Autodesk Inventor part; units mm, degrees
ref_plane "YZ Plane" through (0, 0, 0) normal (1, 0, 0) x (0, 1, 0)
ref_plane "XZ Plane" through (0, 0, 0) normal (0, 1, 0) x (-1, 0, 0)
ref_plane "XY Plane" through (0, 0, 0) normal (0, 0, 1) x (1, 0, 0)
sketch "スケッチ2" plane through (0, 0, 0) normal (0, 1, 0) x (-1, 0, 0)
  line L0 (-6, 0) -> (-6, 5)
  line L1 (-6, 5) -> (-10, 5)
  line L2 (-10, 5) -> (-10, 11.5)
  line L3 (-10, 11.5) -> (-6, 11.5)
  line L4 (-6, 11.5) -> (-6, 12.5)
  line L5 (-6, 12.5) -> (-4, 12.5)
  line L6 (-4, 12.5) -> (-4, 0)
  line L7 (-4, 0) -> (-6, 0)
  line L8 (0, -14.5) -> (0, 17)
  circle A0 centre (0, 0) radius 4 construction
  circle A1 centre (0, 0) radius 10 construction
  circle A2 centre (0, 0) radius 6.7 construction
  dimension "d4" = 4
  dimension "d5" = 6
  dimension "d6" = 10
  dimension "d7" = 12.5
  dimension "d8" = 5
  dimension "d9" = 1
  dimension "d11" = 8
  dimension "d12" = 20
  dimension "d14" = 3.3
revolve "回転1" add sketch "スケッチ2" angle 360 about axis through (0, 0, -10) along (0, 0, 1)
mirror "ミラー1" about plane through (6, 0, 0) normal (0, 0, -1) of "回転1"
properties part number "POMベアリング" material "アセタール樹脂、白"
Build history of the part. All positions in model axes, mm. A direction names the side the tool comes from. Round coordinates to 2 decimals unless told otherwise and drop trailing zeros. Loops run counter-clockwise (first coordinate to the right, second up) from the corner with the lowest first, then second, coordinate; pieces in that order, holes last. Notation, with made-up numbers: (14.25, 33) -> (21.25, 33) arc R5 cw to (21.25, 41) -> close; hole circle Ø9 at (76.25, -10). An arc over 180 degrees is marked (long way). Answer in a Markdown table with one row per item.
Item 1: Pin check, flat tips, straight feed: pin 1 (1.5 mm diameter, centred on x = -7.5, z = -5, fed in from -Y); pin 2 (1.5 mm diameter, centred on x = 1.5, z = 9.5, fed in from +Y); pin 3 (2 mm diameter, centred on x = -2, z = -3, fed in from -Y); pin 4 (7 mm diameter, centred on x = 0, y = 0, fed in from +Z). Stop position of each tip, or through.
Answers below:
| item | result |
|---|---|
| pin 1 | stops at y = -7.38 |
| pin 2 | stops at y = 9.97 |
| pin 3 | stops at y = -5.92 |
| pin 4 | passes through |
Item 2: Mould opens along Z. For faces 1 (the flat face through (7, 0, 5)), 2 (the cylindrical face through (-0.867, -3.905, 0.175)), 3 (the flat face through (-1.42, -3.92, 12.5)) say: +Z half, -Z half, draft (parallel to the pull), parting line (faces both ways), or undercut.
Answers below:
| item | result |
|---|---|
| face 1 | undercut |
| face 2 | draft |
| face 3 | +Z half |
Item 3: Saw through at A-A (y = 0). Write the cut outline in (x, z), and give its area (3 significant figures).
Answers below:
| item | result |
|---|---|
| outline | (-10, -11.5) -> (-6, -11.5) -> (-6, -12.5) -> (-4, -12.5) -> (-4, 12.5) -> (-6, 12.5) -> (-6, 11.5) -> (-10, 11.5) -> (-10, 5) -> (-6, 5) -> (-6, -5) -> (-10, -5) -> close; (4, -12.5) -> (6, -12.5) -> (6, -11.5) -> (10, -11.5) -> (10, -5) -> (6, -5) -> (6, 5) -> (10, 5) -> (10, 11.5) -> (6, 11.5) -> (6, 12.5) -> (4, 12.5) -> close |
| area | 204 mm² |
Item 4: Saw through at C-C (z = 10.5). Write the cut outline in (x, y), and give its area (3 significant figures).
Answers below:
| item | result |
|---|---|
| outline | circle Ø20 at (0, 0); hole circle Ø8 at (0, 0) |
| area | 264 mm² |
Item 5: Drill centre lines: L1, parallel to Z at x = 8, y = 1; L2, parallel to Y at x = 0, z = -5.25; L3, parallel to Y at x = 0, z = 1.5. Where is each one in solid material? Low to high. Write a range as [from, to].
Answers below:
| item | result |
|---|---|
| L1 | z = [-11.5, -5], [5, 11.5] |
| L2 | y = [-10, -4], [4, 10] |
| L3 | y = [-6, -4], [4, 6] |
Item 6: Which spindle directions (+Z, -Z, +X, -X, +Y, -Y) get a long thin tool onto all of the face, cutting with end or side? Do faces 4 (the cylindrical face through (-6, 0, -12)), 5 (the cylindrical face through (-6, 0, 0)), 6 (the flat face through (1.42, -3.92, -12.5)), 7 (the cylindrical face through (-6, 0, 12)), 8 (the cylindrical face through (-2.17, -9.76, 8.3)). Say none if no direction does.
Answers below:
| item | result |
|---|---|
| face 4 | -Z |
| face 5 | none |
| face 6 | -Z, +X, -X, +Y, -Y |
| face 7 | +Z |
| face 8 | +Z, -Z |
Item 7: Saw through at D-D (x = 8). Write the cut outline in (y, z), and give its area (3 significant figures).
Answers below:
| item | result |
|---|---|
| outline | (-6, -11.5) -> (6, -11.5) -> (6, -5) -> (-6, -5) -> close; (-6, 5) -> (6, 5) -> (6, 11.5) -> (-6, 11.5) -> close |
| area | 156 mm² |
